Model file for the job. Use its own axes, mm. Round coordinates to 2 decimals unless told otherwise and drop trailing zeros. Loops run counter-clockwise (first coordinate to the right, second up) from the corner with the lowest first, then second, coordinate; pieces in that order, holes last. Notation, with made-up numbers: M -38,-3 L -20,-3 A15 ccw -20,25 Z; hole C -23,3 d5. An arc over 180 degrees is marked long. Use a Markdown table: item, result. Add a question column.
Q1. Pin check, flat tips, straight feed: pin 1 (0.9 mm diameter, centred on x = -1.5, y = 2, fed in from -Z); pin 2 (1.5 mm diameter, centred on x = 87.5, y = 1, fed in from -Z); pin 3 (1.5 mm diameter, centred on y = 2, z = -281.5, fed in from +X). Stop position of each tip, or through.
Q2. Cut at A-A (z = -230). Give the cut face in (x, y), plus the area to 3 significant figures.
Q3. Probe line 1 (Z direction, x = 136.5, y = 2.4); line 2 (X direction, y = 2.6, z = -94); line 3 (X direction, y = 0.65, z = -264). List the from-to ranges inside material, lowest first. Write a range as from..to.
from build123d import *

# Parameters (mm, degrees)
SALIENTE_EXTRUIR1_DEPTH = 3


with BuildPart() as part:
    # Croquis1 → Saliente-Extruir1 (new body)
    with BuildSketch(Plane(origin=(0, 0, 0), x_dir=(1, 0, 0), z_dir=(0, 1, 0))):
        Polygon((0, 0), (200, 0), (200, 20), (203.1, 20), (203.1, 40), (200, 40), (200, 60), (203.1, 60), (203.1, 80), (200, 80), (200, 100), (203.1, 100), (203.1, 120), (200, 120), (200, 140), (203.1, 140), (203.1, 160), (200, 160), (200, 180), (203.1, 180), (203.1, 200), (200, 200), (200, 220), (203.1, 220), (203.1, 240), (200, 240), (200, 260), (203.1, 260), (203.1, 280), (200, 280), (200, 283.1), (180, 283.1), (180, 280), (160, 280), (160, 283.1), (140, 283.1), (140, 280), (120, 280), (120, 283.1), (100, 283.1), (100, 280), (80, 280), (80, 283.1), (60, 283.1), (60, 280), (40, 280), (40, 283.1), (20, 283.1), (20, 280), (0, 280), (0, 260), (-3.1, 260), (-3.1, 240), (0, 240), (0, 220), (-3.1, 220), (-3.1, 200), (0, 200), (0, 180), (-3.1, 180), (-3.1, 160), (0, 160), (0, 140), (-3.1, 140), (-3.1, 120), (0, 120), (0, 100), (-3.1, 100), (-3.1, 80), (0, 80), (0, 60), (-3.1, 60), (-3.1, 40), (0, 40), (0, 20), (-3.1, 20), (-3.1, 0), align=None)
    extrude(amount=SALIENTE_EXTRUIR1_DEPTH)


solid = part.part
Checked values:
| question | item | result |
|---|---|---|
| 1 | pin 1 | stops at z = -260 |
| 1 | pin 2 | stops at z = -280 |
| 1 | pin 3 | stops at x = 200 |
| 2 | outline | M 0,0 L 203.1,0 L 203.1,3 L 0,3 Z |
| 2 | area | 609 mm^2 |
| 3 | line 1 | z = -280..0 |
| 3 | line 2 | x = -3.1..200 |
| 3 | line 3 | x = 0..203.1 |
